Design review of the part built by this model. Coordinates are the model's own, in mm. A direction names the side the tool comes from. Round coordinates to 2 decimals unless told otherwise and drop trailing zeros. Order: outer loops, then holes, each group sorted by start corner. A loop starts at its lowest first (then second) coordinate and runs counter-clockwise, first axis right, second up. Notation, with made-up numbers: M 19.25,45.5 L 28.25,45.5 A26 cw 28.25,77.5 Z; hole C 41.5,83.25 d2. An arc over 180 degrees is marked long. Write item = value, one per line. Start each with the question number.
Autodesk Fusion 360 part; units mm, degrees
sketch "Sketch1" plane through (0, 0, 0) normal (0, 0, 1) x (1, 0, 0)
  line L0 (0, 20) -> (0, 0)
  line L1 (0, 0) -> (0, 0)
  line L2 (3, 3) -> (3, 7.9338)
  line L3 (9, 13.9338) -> (12, 13.9338)
  line L4 (18, 7.9338) -> (18, 1.5)
  line L5 (19.5, 0) -> (19.4638, 0)
  line L6 (20.9638, 1.5) -> (20.9638, 11.9338)
  line L7 (15.9638, 16.9338) -> (3, 16.9338)
  line L8 (3, 16.9338) -> (3, 20)
  line L9 (3, 20) -> (0, 20)
  arc A0 (20.9638, 11.9338) -> (15.9638, 16.9338) centre (15.9638, 11.9338) ccw
  arc A1 (18, 7.9338) -> (12, 13.9338) centre (12, 7.9338) ccw
  arc A2 (18, 1.5) -> (19.5, 0) centre (19.5, 1.5) ccw
  arc A3 (19.4638, 0) -> (20.9638, 1.5) centre (19.4638, 1.5) ccw
  arc A4 (9, 13.9338) -> (3, 7.9338) centre (9, 7.9338) ccw
  arc A5 (0, 0) -> (3, 3) centre (0, 3) ccw
  dimension "d1" = 5
  dimension "d2" = 6
  dimension "d3" = 1.5
  dimension "d4" = 1.5
  dimension "d5" = 3
  dimension "d6" = 3
  dimension "d7" = 2.9638
  dimension "d9" = 6
  dimension "d10" = 3
  dimension "d11" = 15
  dimension "d13" = 20
extrude "Extrude1" add sketch "Sketch1" along normal blind 5
extrude "Extrude2" add 1 faces at (1.0204, 9.5959, 5) along direction (0, 0, 1) blind 40
(1) Consider section B-B, the plane y = 10.75. Write out the cut boundary in (x, z).
(2) For line 1 along X through (y, z) = (6.75, 5); line 2 along X through (y, z) = (19, 23.5); line 3 along Y through (x, z) = (11.5, 29), list the stretches that pass through material, from the lowest coordinate up. Write a range as [from, to].
(3) Insertion check: pin 1 (6 mm diameter, centred on x = 12, z = 33.5, fed in from +Y); pin 2 (8 mm diameter, centred on y = 17.5, z = 33, fed in from +X); pin 3 (2 mm diameter, centred on x = 16.5, z = 22, fed in from -Y). Each pin has a flat end and moves straight along its axis. Give the tip position at first contact, or say it passes through.
(4) Consider section A-A, the plane y = 7. Write out the cut boundary in (x, z).
(5) For faces 1 (the face through (10, 16.934, 22)), 2 (the face through (20.964, 7, 22)), 3 (the face through (16.2, 12.22, 22.18)), list the 3-axis set-ups (+Z, -Z, +X, -X, +Y, -Y) from which the entire face can be reached by the end or side of a thin tool; tool diameter is ignored.
(6) Consider section D-D, the plane x = 9.75. Write out the cut boundary in (y, z), then the cut area to 3 significant figures.
(7) Draft analysis for pull direction X (two halves, no side actions). For faces 4 (the face through (10, 15, 45)), 5 (the face through (18.44, 0.44, 22.18)), 6 (the face through (19.46, 15.51, 22.18)), state which applies: pulls with the +X half, pulls with the -X half, needs draft (parallel to the pull), parting line crosses it, or undercut.
Completed:
q1.outline = M 0,0 L 3.7,0 L 3.7,45 L 0,45 Z; M 17.3,0 L 20.96,0 L 20.96,45 L 17.3,45 Z
q2.line_1 = [0, 3], [18, 20.96]
q2.line_2 = [0, 3]
q2.line_3 = [13.93, 16.93]
q3.pin_1 = 16.93
q3.pin_2 = 20.71
q3.pin_3 = 10.33
q4.outline = M 0,0 L 3,0 L 3,45 L 0,45 Z; M 18,0 L 20.96,0 L 20.96,45 L 18,45 Z
q5.face_1 = +Z, -Z, +X, +Y
q5.face_2 = +Z, -Z, +X, +Y, -Y
q5.face_3 = +Z, -Z, -Y
q6.outline = M 13.93,0 L 16.93,0 L 16.93,45 L 13.93,45 Z
q6.area = 135 mm2
q7.face_4 = needs draft
q7.face_5 = undercut
q7.face_6 = pulls with the +X half
